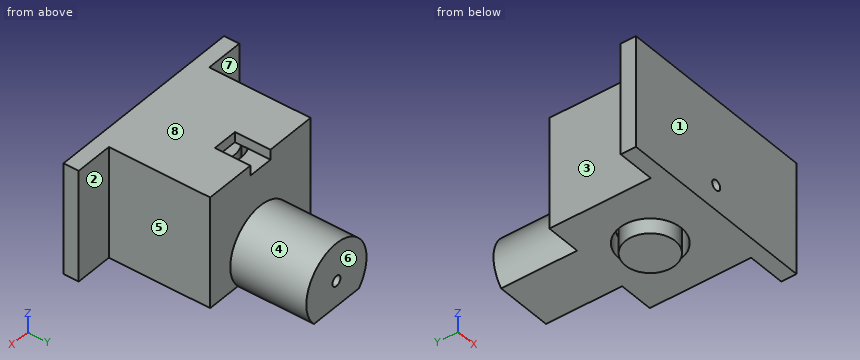
Autodesk Inventor part; units mm, degrees
ref_plane "YZ Plane" through (0, 0, 0) normal (1, 0, 0) x (0, 1, 0)
ref_plane "XZ Plane" through (0, 0, 0) normal (0, 1, 0) x (-1, 0, 0)
ref_plane "XY Plane" through (0, 0, 0) normal (0, 0, 1) x (1, 0, 0)
sketch "Sketch1" plane through (0, 0, 0) normal (0, 0, 1) x (1, 0, 0)
  circle A0 centre (0, 0) radius 6.1
  line L0 (-12.5, -10) -> (12.5, -10)
  line L1 (12.5, -10) -> (12.5, 10)
  line L2 (12.5, 10) -> (-12.5, 10)
  line L3 (-12.5, 10) -> (-12.5, -10)
  line L4 (-12.5, -10) -> (12.5, 10) construction
  line L5 (12.5, -10) -> (-12.5, 10) construction
  dimension "d0" = 12.2
  dimension "d1" = 25
  dimension "d2" = 20
extrude "Extrusion1" add sketch "Sketch1" along normal blind 20
sketch "Sketch2" plane through (-12.5, 10, 0) normal (0, 1, 0) x (1, 0, 0)
  line L0 (0, 0) -> (0, -20) construction
  line L1 (25, -20) -> (0, -20) construction
  line L2 (0, 0) -> (25, -20) construction
  line L3 (0, -20) -> (25, 0) construction
  circle A0 centre (12.5, -10) radius 1
  point P0 (12.5, 0)
  dimension "d5" = 2
extrude "Extrusion2" cut sketch "Sketch2" against normal blind 100
sketch "Sketch3" plane through (-12.5, 10, 0) normal (0, 1, 0) x (1, 0, 0)
  circle A0 centre (12.5, -10) radius 1
  line L0 (25, 0) -> (0, 0)
  line L1 (0, 0) -> (0, -20)
  line L2 (25, -20) -> (0, -20)
  line L3 (25, 0) -> (25, -20)
  circle A1 centre (12.5, -10) radius 7.5
  point P0 (12.5, 0)
  dimension "d8" = 15
extrude "Extrusion3" add sketch "Sketch3" along normal blind 15 contours A1
sketch "Sketch4" plane through (-12.5, -10, 0) normal (0, -1, 0) x (1, 0, 0)
  line L0 (32.5, 25) -> (-7.5, 25)
  line L1 (-7.5, 25) -> (-7.5, -5)
  line L2 (-7.5, -5) -> (32.5, -5)
  line L3 (32.5, -5) -> (32.5, 25)
  circle A0 centre (12.5, 10) radius 1
  line L4 (32.5, 25) -> (-7.5, -5) construction
  line L5 (-7.5, 25) -> (32.5, -5) construction
  point P0 (12.5, 0)
  dimension "d11" = 30
  dimension "d12" = 40
extrude "Extrusion4" add sketch "Sketch4" along normal blind 3
thicken "Thicken1" operation add thickness 5 both sides no extend neighbours yes toward (0, 0, 1) faces at (-10.3667, 0, 20)
sketch "Sketch5" plane through (-20, -10, 25) normal (0, 0, 1) x (1, 0, 0)
  line L0 (7.5, 20) -> (7.5, 0)
  line L1 (0, -3) -> (40, -3)
  line L2 (7.5, 20) -> (17.5, 20)
  line L3 (17.5, 20) -> (17.5, -3)
  line L4 (17.5, -3) -> (7.5, -3)
  line L5 (7.5, -3) -> (7.5, 20)
  line L6 (32.5, 0) -> (32.5, 20)
  line L7 (32.5, 20) -> (22.5, 20)
  line L8 (22.5, 20) -> (22.5, -3)
  line L9 (22.5, -3) -> (32.5, -3)
  line L10 (32.5, -3) -> (32.5, 20)
  line L11 (32.5, 0) -> (32.5, 20)
  line L12 (32.5, 20) -> (7.5, 20)
  line L13 (7.5, 20) -> (7.5, 0)
  line L14 (7.5, 0) -> (0, 0)
  line L15 (0, 0) -> (0, -3)
  line L16 (40, -3) -> (0, -3)
  line L17 (40, 0) -> (40, -3)
  line L18 (40, 0) -> (32.5, 0)
  circle A0 centre (20, 10) radius 6.1
  line L19 (17.5, 13) -> (22.5, 13)
  point P0 (22.5, -3)
  dimension "d17" = 10
  dimension "d18" = 10
  dimension "d28" = 3
extrude "Extrusion5" add sketch "Sketch5" along normal blind 2 contours L2 L3 A0 L1 L5 L0 | L5 L1 L15 L14 | L3 A0 | L7 L6 L10 L1 L8 A0 | L3 A0 L8 L1 | L19 L8 A0 L3 | A0 L8 | L18 L17 L1 L10 picked at (20, 9.9667)
sketch "Sketch6" plane through (20, -10, -5) normal (0, 0, -1) x (-1, 0, 0)
  line L0 (-13.3468, 43.0165) -> (63.7046, 43.0165)
  line L1 (63.7046, 43.0165) -> (63.7046, -16.6019)
  line L2 (63.7046, -16.6019) -> (-13.3468, -16.6019)
  line L3 (-13.3468, -16.6019) -> (-13.3468, 43.0165)
  point P0 (20, 10)
extrude "Extrusion6" cut sketch "Sketch6" against normal blind 10
sketch "Sketch7" plane through (-20, -10, 25) normal (0, 0, -1) x (-1, 0, 0)
  circle A0 centre (-20, 10) radius 4.9
  dimension "d23" = 9.8
extrude "Extrusion7" add sketch "Sketch7" along normal blind 22
sketch "Sketch8" plane through (-12.5, 25, 0) normal (0, 1, 0) x (1, 0, 0)
  circle A0 centre (12.5, -10) radius 1
  point P0 (12.5, 0)
extrude "Extrusion8" cut sketch "Sketch8" against normal blind 100
properties part number "New_hinge_template"
Check sheet for the modelled part. Datum: model origin and axes. Units: mm. Face numbers are marked on the shaded views. A direction names the side the tool comes from. Coordinates: 2 decimals unless noted, no trailing zeros. Loops run counter-clockwise (first coordinate to the right, second up) from the corner with the lowest first, then second, coordinate; pieces in that order, holes last.
1) Sectioned sample at C-C (x = 0). Record the boundary of the cut face in (y, z).
2) Gauge pin test, flat ends, axial feed: pin 1 (1 mm diameter, centred on x = 0, y = 4, fed in from +Z); pin 2 (6 mm diameter, centred on y = -1.5, z = 15.5, fed in from +X); pin 3 (6 mm diameter, centred on y = 5, z = 12, fed in from -X). Record the tip position at first contact, or that the pin passes through.
3) Sectioned sample at A-A (z = 19.5). Record the boundary of the cut face in (x, y).
4) Access from +Z, -Z, +X, -X, +Y, -Y to the whole of each face (thin tool, end or side, straight path). Record for the marked faces 4, 5, 6, 7 and 8.
5) Release check for a two-part mould opening along Y. For the marked faces 1, 2 and 3 record: released by +Y, released by -Y, zero draft, split by the parting line, or undercut.
6) Sectioned sample at B-B (y = 9.5). Record the boundary of the cut face in (x, z).
7) Sectioned sample at D-D (z = 10). Record the boundary of the cut face in (x, y).
8) Material ranges on probe 1 along Y at (x, z) = (2.5, 15); probe 2 along Z at (x, y) = (0, 2); probe 3 along X at (y, z) = (0.5, 10), recorded low to high.
Check sheet entries:
1. outline: (-13, 5) - (-6.1, 5) - (-6.1, 9) - (-13, 9) - close; (-13, 11) - (-6.1, 11) - (-6.1, 25) - (-4.9, 25) - (-4.9, 11) - (4.9, 11) - (4.9, 25) - (3, 25) - (3, 27) - (-13, 27) - close; (-4.9, 3) - (4.9, 3) - (4.9, 9) - (-4.9, 9) - close; (6.1, 5) - (25, 5) - (25, 9) - (6.1, 9) - close; (6.1, 11) - (25, 11) - (25, 17.5) - (10, 17.5) - (10, 25) - (6.1, 25) - close
2. pin 1: stops at z = 25
2. pin 2: stops at x = 12.5
2. pin 3: stops at x = -12.5
3. outline: (-20, -13) - (20, -13) - (20, -10) - (12.5, -10) - (12.5, 10) - (-12.5, 10) - (-12.5, -10) - (-20, -10) - close; circle Ø9.8 at (0, 0); hole circle Ø12.2 at (0, 0)
4. face 4: +Y
4. face 5: +Z, -Z, +X, +Y
4. face 6: +Z, -Z, +X, -X, +Y
4. face 7: +Z, -Z, -X, +Y
4. face 8: +Z, +X, -X, +Y, -Y
5. face 1: released by -Y
5. face 2: released by +Y
5. face 3: zero draft
6. outline: (-12.5, 5) - (12.5, 5) - (12.5, 27) - (2.5, 27) - (2.5, 25) - (-2.5, 25) - (-2.5, 27) - (-12.5, 27) - close; hole circle Ø2 at (0, 10)
7. outline: (-20, -13) - (-1, -13) - (-1, -6.02) arc R6.1 cw to (-1, 6.02) - (-1, 25) - (-7.5, 25) - (-7.5, 10) - (-12.5, 10) - (-12.5, -10) - (-20, -10) - close; (-1, -4.8) - (-1, 4.8) arc R4.9 ccw to start; (1, -13) - (20, -13) - (20, -10) - (12.5, -10) - (12.5, 10) - (7.5, 10) - (7.5, 25) - (1, 25) - (1, 6.02) arc R6.1 cw to (1, -6.02) - close; (1, -4.8) arc R4.9 ccw to (1, 4.8) - close
8. probe 1: y = -13 to -5.56, -4.21 to 4.21, 5.56 to 25
8. probe 2: z = 3 to 9, 11 to 27
8. probe 3: x = -12.5 to -6.08, -4.87 to -1, 1 to 4.87, 6.08 to 12.5
